The listing builds one solid part. Answer for the finished solid, in the listing's coordinates (mm). A direction names the side the tool comes from. Give positions to 0.01 mm unless a question says otherwise; leave off trailing zeros. Order: outer loops, then holes, each group sorted by start corner. A loop starts at its lowest first (then second) coordinate and runs counter-clockwise, first axis right, second up. Notation, with made-up numbers: (-1, 6) - (18, 6) arc R13 cw to (18, 11) - close; hole circle Ø11 at (78, -36.5). An arc over 180 degrees is marked (long way). Answer as CSV lines item,"result". Start each with the question number.
1. Section D-D on x = 4.75 is taken. Give the vertices of the cut face in (y, z) (3 decimals).
2. Determine the mould class of faces 3 (the flat face through (11, 2, 2)), 4 (the flat face through (0, -8, 3)), 5 (the cylindrical face through (3.905, -1.557, 1.565)), 6 (the cylindrical face through (21.861, -2.564, 1.565)) for opening direction X: +X half, -X half, draft (parallel to the pull), parting line (faces both ways), or undercut.
3. Section A-A on x = 11.5 is taken. Give the vertices of the cut face in (y, z) (3 decimals).
4. Section C-C on z = 2.25 is taken. Give the vertices of the cut face in (x, y) (3 decimals), and give its area (3 significant figures).
5. Section B-B on y = -2 is taken. Give the vertices of the cut face in (x, z) (3 decimals), and give its area (3 significant figures).
6. Consider line 1 along X through (y, z) = (-3.25, 1.5); line 2 along Y through (x, z) = (20.5, 1.4) (3 decimals); line 3 along X through (y, z) = (-2.5, 2.5). Determine where each line is inside the solid, lowest interval first. Write a range as [from, to].
7. Flat-ended cylindrical pins translate along their axes: pin 1 (4 mm diameter, centred on x = 6.5, z = 5, fed in from +Y); pin 2 (6 mm diameter, centred on x = 20.5, z = 7.5, fed in from +Y); pin 3 (5 mm diameter, centred on x = 17, y = -2.5, fed in from +Z) (3 decimals); pin 4 (2 mm diameter, centred on x = 20, z = 4.5, fed in from +Y). Find the tip coordinate at first contact, or state that the pin passes through.
8. Which of the six approach directions +Z, -Z, +X, -X, +Y, -Y give full straight-line access (tool end or side, diameter ignored) to faces 1 (the flat face through (23, -8, 3)), 2 (the flat face through (11, -3, 3.175))?
from build123d import *

# Parameters (mm, degrees)
SKETCH1_W             = 23
SKETCH1_H             = 10
SKETCH1_R             = 1.4732
SKETCH1_H_2           = 3.175
SKETCH1_H_3           = 2
BOSS_EXTRUDE1_DEPTH   = 3.175
BOSS_EXTRUDE2_START   = 3.175
SKETCH1_3_W           = 23
SKETCH1_3_H           = 3.175
BOSS_EXTRUDE2_DEPTH   = 9
F_8_32_TAPPED_HOLE1_D = 3.4544
FILLET1_R             = 1


with BuildPart() as part:
    # Sketch1 → Boss-Extrude1 (new body)
    # profile 1 of 3: a face of its own
    with BuildSketch(Plane.XY):
        with Locations((11.5, -5)):
            Rectangle(SKETCH1_W, SKETCH1_H)
        with Locations((2.5, -2)):
            Circle(SKETCH1_R, mode=Mode.SUBTRACT)
        with Locations((20.5, -2)):
            Circle(SKETCH1_R, mode=Mode.SUBTRACT)
    # profile 2 of 3: a face of its own
    with BuildSketch(Plane.XY):
        with Locations((11.5, -11.5875)):
            Rectangle(SKETCH1_W, SKETCH1_H_2)
    # profile 3 of 3: a face of its own
    with BuildSketch(Plane.XY):
        with Locations((11.5, 1)):
            Rectangle(SKETCH1_W, SKETCH1_H_3)
    extrude(amount=BOSS_EXTRUDE1_DEPTH)

    # Sketch1<3> → Boss-Extrude2 (add)
    with BuildSketch(Plane.XY.offset(BOSS_EXTRUDE2_START)):
        with Locations((11.5, -11.5875)):
            Rectangle(SKETCH1_3_W, SKETCH1_3_H)
    extrude(amount=BOSS_EXTRUDE2_DEPTH)

    # #8-32 Tapped Hole1 (through all)
    with Locations(Plane(origin=(11.5, -10, 8.175), x_dir=(1, 0, 0), z_dir=(0, 1, 0))):
        with Locations((0, 0)):
            Hole(F_8_32_TAPPED_HOLE1_D / 2)

    # Fillet1
    fillet1_edges = [part.edges().sort_by_distance(p)[0] for p in [
        (0, 2, 1.5875),
        (23, 2, 1.5875),
        (0, -11.5875, 12.175),
        (11.5, -10, 3.175),
        (23, -11.5875, 12.175),
        (11.5, -13.175, 0),
    ]]
    fillet(fillet1_edges, radius=FILLET1_R)


solid = part.part
Checks:
1,outline,"(-13.175, 1) arc R1 ccw to (-12.175, 0) - (2, 0) - (2, 3.175) - (-9, 3.175) arc R1 cw to (-10, 4.175) - (-10, 12.175) - (-13.175, 12.175) - close"
2,face 3,"draft"
2,face 4,"-X half"
2,face 5,"undercut"
2,face 6,"undercut"
3,outline,"(-13.175, 1) arc R1 ccw to (-12.175, 0) - (2, 0) - (2, 3.175) - (-9, 3.175) arc R1 cw to (-10, 4.175) - (-10, 6.448) - (-13.175, 6.448) - close; (-13.175, 9.902) - (-10, 9.902) - (-10, 12.175) - (-13.175, 12.175) - close"
4,outline,"(0, -13.175) - (23, -13.175) - (23, 1) arc R1 ccw to (22, 2) - (1, 2) arc R1 ccw to (0, 1) - close; hole circle Ø2.946 at (2.5, -2); hole circle Ø2.946 at (20.5, -2)"
4,area,"335 mm²"
5,outline,"(0, 0) - (1.027, 0) - (1.027, 3.175) - (0, 3.175) - close; (3.973, 0) - (19.027, 0) - (19.027, 3.175) - (3.973, 3.175) - close; (21.973, 0) - (23, 0) - (23, 3.175) - (21.973, 3.175) - close"
5,area,"54.3 mm²"
6,line 1,"x = [0, 1.72], [3.28, 19.72], [21.28, 23]"
6,line 2,"y = [-13.175, -3.473], [-0.527, 2]"
6,line 3,"x = [0, 1.11], [3.89, 19.11], [21.89, 23]"
7,pin 1,"stops at y = 2"
7,pin 2,"stops at y = -10"
7,pin 3,"stops at z = 3.175"
7,pin 4,"stops at y = -9.74"
8,face 1,"+Z, -Z, +X, +Y, -Y"
8,face 2,"+Z, +X, -X, +Y"
